```python
from build123d import *

# Parameters (mm, degrees)
SPACER_DEPTH       = 20
HOLE_R             = 1.25
BLIND_HOLE_DEPTH   = 6.5
HOLE_CHAMFER_SIZE  = 0.25
SHAFT_R            = 1.5
MAIL_SHAFT_DEPTH   = 6.5
SHAFT_CHAMFER_SIZE = 0.25


with BuildPart() as part:
    # Profile → SPACER (new body)
    with BuildSketch(Plane(origin=(0, 0, 0), x_dir=(1, 0, 0), z_dir=(0, 1, 0))):
        Polygon((-2.4, -1.385640646), (0, -2.771281292), (2.4, -1.385640646), (2.4, 1.385640646), (0, 2.771281292), (-2.4, 1.385640646), align=None)
    extrude(amount=SPACER_DEPTH)

    # HOLE → BLIND_HOLE (cut)
    with BuildSketch(Plane(origin=(0, 20, 0), x_dir=(1, 0, 0), z_dir=(0, 1, 0))):
        with Locations(Location((0, 0, 0), (0, 0, 270))):
            Circle(HOLE_R)
    extrude(amount=-BLIND_HOLE_DEPTH, mode=Mode.SUBTRACT)

    # HOLE_Chamfer
    hole_chamfer_edges = [part.edges().sort_by_distance(p)[0] for p in [
        (0, 20, -1.25),
    ]]
    chamfer(hole_chamfer_edges, length=HOLE_CHAMFER_SIZE)

    # Sketch6 → DRILL_CUT (revolve, cut)
    with BuildSketch(Plane.XY, mode=Mode.PRIVATE) as drill_cut_sk:
        Polygon((0, 13.5), (-1.25, 13.5), (0, 12.748924226), align=None)
    revolve(drill_cut_sk.sketch.rotate(Axis((0, 12.748924226, 0), (0, 1, 0)), 90), axis=Axis((0, 12.748924226, 0), (0, 1, 0)), mode=Mode.SUBTRACT)

    # SHAFT → MAIL_SHAFT (add)
    with BuildSketch(Plane.XZ):
        with Locations(Location((0, 0, 0), (0, 0, 90))):
            Circle(SHAFT_R)
    extrude(amount=MAIL_SHAFT_DEPTH)

    # SHAFT_Chamfer
    shaft_chamfer_edges = [part.edges().sort_by_distance(p)[0] for p in [
        (0, -6.5, -1.5),
    ]]
    chamfer(shaft_chamfer_edges, length=SHAFT_CHAMFER_SIZE)


solid = part.part
```
Work out the finished part from the listing and answer in its coordinate system (mm). A direction names the side the tool comes from. Coordinates: 2 decimals unless noted, no trailing zeros. Loops run counter-clockwise (first coordinate to the right, second up) from the corner with the lowest first, then second, coordinate; pieces in that order, holes last. Notation, with made-up numbers: (42.25, 13) - (97.25, 13) arc R30 cw to (97.25, 51) - close; hole circle Ø7 at (88.25, 16). An arc over 180 degrees is marked (long way). Use a Markdown table: item, result.
Item 1: Find section D-D, the plane y = -4.5. Determine the outline of the cut face in (x, z).
Evaluation:
| item | result |
|---|---|
| outline | circle Ø3 at (0, 0) |
Item 2: Consider probe 1 along X at (y, z) = (16.75, 0); probe 2 along Y at (x, z) = (-1.3, 1.9); probe 3 along X at (y, z) = (7, -1.9). Determine where each line is inside the solid, lowest interval first. Write a range as from..to.
Evaluation:
| item | result |
|---|---|
| probe 1 | x = -2.4..-1.25, 1.25..2.4 |
| probe 2 | y = 0..20 |
| probe 3 | x = -1.51..1.51 |
Item 3: Find section A-A, the plane y = 14.75. Determine the outline of the cut face in (x, z), and give its area (3 significant figures).
Evaluation:
| item | result |
|---|---|
| outline | (-2.4, -1.39) - (0, -2.77) - (2.4, -1.39) - (2.4, 1.39) - (0, 2.77) - (-2.4, 1.39) - close; hole circle Ø2.5 at (0, 0) |
| area | 15.0 mm2 |
Item 4: For faces 1 (the cylindrical face through (-1.22, 16.67, -0.27)), 2 (the flat face through (-1.18, 9.86, -2.09)), 3 (the flat face through (-2, 0, 0)), determine the directions among +Z, -Z, +X, -X, +Y, -Y from which every point of the face is accessible in a straight line to the end or side of a thin tool.
Evaluation:
| item | result |
|---|---|
| face 1 | +Y |
| face 2 | -Z, -X, +Y, -Y |
| face 3 | -Y |
Item 5: Find section B-B, the plane y = 1.5. Determine the outline of the cut face in (x, z), and give its area (3 significant figures).
Evaluation:
| item | result |
|---|---|
| outline | (-2.4, -1.39) - (0, -2.77) - (2.4, -1.39) - (2.4, 1.39) - (0, 2.77) - (-2.4, 1.39) - close |
| area | 20.0 mm2 |
Item 6: The mould has two halves that part along Z. Classify faces 4 (the flat face through (-2, 20, 0)), 5 (the flat face through (1.18, 9.86, 2.09)), 6 (the conical face through (-0.12, 12.87, -0.16)): +Z half, -Z half, draft (parallel to the pull), parting line (faces both ways), or undercut.
Evaluation:
| item | result |
|---|---|
| face 4 | draft |
| face 5 | +Z half |
| face 6 | undercut |
Item 7: Given pin 1 Ø1 at (x, y) = (1.5, 0.5) entering from +Z, flat-ended and moving along its own axis, determine where the tip first touches the part or whether it passes through.
Evaluation:
| item | result |
|---|---|
| pin 1 | stops at z = 2.19 |
Item 8: Find section C-C, the plane z = 2.35. Determine the outline of the cut face in (x, y).
Evaluation:
| item | result |
|---|---|
| outline | (-0.73, 0) - (0.73, 0) - (0.73, 20) - (-0.73, 20) - close |
